Autodesk Inventor part; units mm, degrees
ref_plane "YZ Plane" through (0, 0, 0) normal (1, 0, 0) x (0, 1, 0)
ref_plane "XZ Plane" through (0, 0, 0) normal (0, 1, 0) x (-1, 0, 0)
ref_plane "XY Plane" through (0, 0, 0) normal (0, 0, 1) x (1, 0, 0)
sketch "スケッチ1" plane through (0, 0, 0) normal (0, 1, 0) x (-1, 0, 0)
  line L0 (34, -11) -> (-51, -11)
  line L1 (-51, -11) -> (-51, 11)
  line L2 (-51, 11) -> (34, 11)
  line L3 (34, 11) -> (34, -11)
  line L4 (34, 0) -> (-51, 0) construction
  point P0 (0, 0)
  point P1 (0, 0)
  point P2 (-46, 0)
  dimension "d0" = 22
  dimension "d1" = 85
  dimension "d2" = 5
  dimension "d3" = 46
extrude "押し出し1" add sketch "スケッチ1" along normal blind 12
sketch "スケッチ2" plane through (0, 12, 0) normal (0, 1, 0) x (1, 0, 0)
  line L0 (-34, 11) -> (-34, -11)
  line L1 (51, -11) -> (51, 11)
  line L2 (-34, 0) -> (51, 0)
  line L3 (51, 0) -> (51, 6)
  line L4 (51, 6) -> (-34, 6)
  line L5 (-34, 6) -> (-34, 0)
  line L6 (51, 0) -> (51, -6)
  line L7 (51, -6) -> (-34, -6)
  line L8 (-34, -6) -> (-34, 0)
  point P0 (0, 0)
  point P1 (-34, -6)
  point P2 (-34, 6)
  dimension "d6" = 12
extrude "押し出し2" cut sketch "スケッチ2" against normal blind 7
sketch "スケッチ3" plane through (0, 5, 0) normal (0, 1, 0) x (1, 0, 0)
  point P0 (0, 0)
  point P1 (-4, 0)
  point P2 (46, 0)
  dimension "d9" = 4
  dimension "d10" = 50
hole "穴1" at (-4, 5, 0) at (46, 5, 0) direction (0, -1, 0) diameter 2.459 end through all
sketch "スケッチ4" plane through (-34, 0, -11) normal (-1, 0, 0) x (0, 0, 1)
  line L0 (0, 38.5) -> (22, 38.5)
  line L1 (22, 38.5) -> (22, -21.5)
  line L2 (22, -21.5) -> (0, -21.5)
  line L3 (0, -21.5) -> (0, 38.5)
  line L4 (0, 0) -> (0, 12)
  line L5 (22, 0) -> (22, 12)
  line L6 (0, 12) -> (5, 12) construction
  line L7 (5, 12) -> (17, 5) construction
  line L8 (22, 38.5) -> (0, -21.5) construction
  point P0 (11, 0)
  point P1 (11, 8.5)
  dimension "d18" = 60
extrude "押し出し3" add sketch "スケッチ4" against normal blind 10
sketch "スケッチ5" plane through (-34, 38.5, 11) normal (0, 1, 0) x (1, 0, 0)
  line L0 (0, 22) -> (10, 22)
  line L1 (0, 0) -> (10, 0)
  circle A0 centre (5, 0) radius 2.5
  circle A1 centre (5, 22) radius 2.5
  point P0 (34, 11)
  dimension "d21" = 5
  dimension "d22" = 5
extrude "押し出し4" cut sketch "スケッチ5" against normal through all
properties part number "forkmount" material "ABS プラスチック"
For this review, take the finished solid that the model builds, in its own axes (mm). A direction names the side the tool comes from. Round coordinates to 2 decimals unless told otherwise and drop trailing zeros. Write each loop counter-clockwise with the first axis right and the second up, starting at its lowest first coordinate (ties: lowest second). Pieces come first, ordered by that corner, then holes. Notation, with made-up numbers: (85.5, 34) - (140.5, 34) arc R20 cw to (140.5, 71) - close; hole circle Ø2 at (-12, 79.25). An arc over 180 degrees is marked (long way). Write item = value, one per line. Start each with the question number.
1. For faces 1 (the face through (14, 0, 0)), 2 (the face through (14, 9, 6)), 3 (the face through (14, 12, -8)), 4 (the face through (6, 8, -11)), list the 3-axis set-ups (+Z, -Z, +X, -X, +Y, -Y) from which the entire face can be reached by the end or side of a thin tool; tool diameter is ignored.
2. Consider section D-D on x = -29. State the section outline as (y, z) points, plus the area to 3 significant figures.
3. Consider section C-C on y = -5.5. State the section outline as (x, z) points, plus the area to 3 significant figures.
4. Draft analysis for pull direction Z (two halves, no side actions). For faces 5 (the face through (14, 9, -6)), 6 (the face through (-24, -11, 0)), 7 (the face through (-28.9, 8.9, 8.5)), state which applies: released by +Z, released by -Z, zero draft, split by the parting line, or undercut.
5. Consider section A-A on x = -4. State the section outline as (y, z) points.
6. For pin 1 Ø1.5 at (x, z) = (18, 7.5) entering from +Y; pin 2 Ø6.5 at (y, z) = (23, 3.5) entering from +X; pin 3 Ø1.5 at (x, z) = (46, 0) entering from +Y; pin 4 Ø2 at (x, z) = (22.5, 3.5) entering from +Y, all flat-tipped, find the tip position at first contact; note any pin that passes through.
7. Consider section B-B on z = -3.25. State the section outline as (x, y) points.
8. Wall thickness on L1, parallel to X at y = 1.6, z = 0; L2, parallel to X at y = 19.5, z = 2.5; L3, parallel to Y at x = 40.5, z = -7.75: over which ranges is each line inside the solid? List them lowest first.
Evaluation:
q1.face_1 = +Z, -Z, +X, -Y
q1.face_2 = +X, +Y
q1.face_3 = +Z, -Z, +X, +Y
q1.face_4 = -Z, +X, -X, +Y, -Y
q2.outline = (-21.5, -8.5) - (38.5, -8.5) - (38.5, 8.5) - (-21.5, 8.5) - close
q2.area = 1,020 mm2
q3.outline = (-34, -11) - (-31.5, -11) arc R2.5 cw to (-26.5, -11) - (-24, -11) - (-24, 11) - (-26.5, 11) arc R2.5 cw to (-31.5, 11) - (-34, 11) - close
q3.area = 200 mm2
q4.face_5 = undercut
q4.face_6 = zero draft
q4.face_7 = released by +Z
q5.outline = (0, -11) - (12, -11) - (12, -6) - (5, -6) - (5, -1.23) - (0, -1.23) - close; (0, 1.23) - (5, 1.23) - (5, 6) - (12, 6) - (12, 11) - (0, 11) - close
q6.pin_1 = 12
q6.pin_2 = -24
q6.pin_3 = through
q6.pin_4 = 5
q7.outline = (-34, -21.5) - (-24, -21.5) - (-24, 0) - (51, 0) - (51, 5) - (-24, 5) - (-24, 38.5) - (-34, 38.5) - close
q8.L1 = -34 to -5.23, -2.77 to 44.77, 47.23 to 51
q8.L2 = -34 to -24
q8.L3 = 0 to 12
